from build123d import *

# Parameters (mm, degrees)
SKETCH1_W           = 47.117
SKETCH1_H           = 30.226
BOSS_EXTRUDE1_DEPTH = 23.8506
SKETCH4_W           = 44.069
SKETCH4_H           = 27.178
CUT_EXTRUDE1_DEPTH  = 61.847957117
SKETCH5_R           = 11.43
BOSS_EXTRUDE3_DEPTH = 44.069
SKETCH3_R           = 1.4986
CUT_EXTRUDE2_DEPTH  = 2.54
CUT_EXTRUDE3_START  = -2.54
SKETCH6_R           = 1.4986
CUT_EXTRUDE3_DEPTH  = 2.54
SKETCH2_R           = 1.4478
CUT_EXTRUDE4_DEPTH  = 61.847957117
SKETCH7_R           = 4.1783
CUT_EXTRUDE5_DEPTH  = 32.1564
CHAMFER1_SIZE       = 4.064
CHAMFER1_SIZE2      = 2.346351494


with BuildPart() as part:
    # Sketch1 → Boss-Extrude1 (new body)
    with BuildSketch(Plane.XY):
        with Locations((23.5585, 15.113)):
            Rectangle(SKETCH1_W, SKETCH1_H)
    extrude(amount=BOSS_EXTRUDE1_DEPTH)

    # Sketch4 → Cut-Extrude1 (cut, through all)
    with BuildSketch(Plane.XY.offset(23.8506)):
        with Locations((23.5585, 15.113)):
            Rectangle(SKETCH4_W, SKETCH4_H)
    extrude(amount=-CUT_EXTRUDE1_DEPTH, mode=Mode.SUBTRACT)

    # Sketch5 → Boss-Extrude3 (add)
    with BuildSketch(Plane(origin=(1.524, 0, 0), x_dir=(0, 0, -1), z_dir=(1, 0, 0))):
        with Locations(Location((-11.9253, 15.113, 0), (0, 0, 180))):
            Circle(SKETCH5_R)
    extrude(amount=BOSS_EXTRUDE3_DEPTH)

    # Sketch3 → Cut-Extrude2 (cut)
    with BuildSketch(Plane(origin=(0, 30.226, 0), x_dir=(1, 0, 0), z_dir=(0, 1, 0))):
        with Locations(Location((10.8585, -11.9253, 0), (0, 0, 270))):
            Circle(SKETCH3_R)
        with Locations(Location((36.2585, -11.9253, 0), (0, 0, 270))):
            Circle(SKETCH3_R)
    extrude(amount=-CUT_EXTRUDE2_DEPTH, mode=Mode.SUBTRACT)

    # Sketch6 → Cut-Extrude3 (cut)
    with BuildSketch(Plane.XZ.offset(CUT_EXTRUDE3_START)):
        with Locations(Location((15.9766, 19.812, 0), (0, 0, 270))):
            Circle(SKETCH6_R)
        with Locations(Location((10.8585, 11.9253, 0), (0, 0, 90))):
            Circle(SKETCH6_R)
        with Locations(Location((36.5506, 4.0386, 0), (0, 0, 270))):
            Circle(SKETCH6_R)
    extrude(amount=CUT_EXTRUDE3_DEPTH, mode=Mode.SUBTRACT)

    # Sketch2 → Cut-Extrude4 (cut, through all)
    with BuildSketch(Plane(origin=(47.117, 0, 0), x_dir=(0, 0, -1), z_dir=(1, 0, 0))):
        with Locations((-11.9253, 15.113)):
            Circle(SKETCH2_R)
    extrude(amount=-CUT_EXTRUDE4_DEPTH, mode=Mode.SUBTRACT)

    # Sketch7 → Cut-Extrude5 (cut)
    with BuildSketch(Plane.ZY):
        with Locations((11.9253, 15.113)):
            Circle(SKETCH7_R)
    extrude(amount=-CUT_EXTRUDE5_DEPTH, mode=Mode.SUBTRACT)

    # Chamfer1
    chamfer1_edges = [part.edges().sort_by_distance(p)[0] for p in [
        (32.1564, 15.113, 7.747),
    ]]
    chamfer1_side = [part.faces().sort_by_distance(p)[0] for p in [
        (16.0782, 15.113, 7.747),
    ]]
    chamfer(chamfer1_edges, length=CHAMFER1_SIZE, length2=CHAMFER1_SIZE2, reference=chamfer1_side[0])


solid = part.part
Part model, mm, in its own coordinate system. A direction names the side the tool comes from. Coordinates: 2 decimals unless noted, no trailing zeros. Order: outer loops, then holes, each group sorted by start corner. A loop starts at its lowest first (then second) coordinate and runs counter-clockwise, first axis right, second up. Notation, with made-up numbers: M 49.5,26.25 L 88.5,26.25 A20 cw 88.5,47.25 Z; hole C 62,-16.75 d2. An arc over 180 degrees is marked long. Use a Markdown table: item, result.
(1) Cut at D-D on z = 4.75. Write the cut outline in (x, y), then the cut area to 3 significant figures.
A:
| item | result |
|---|---|
| outline | M 0,0 L 35.23,0 L 35.23,1.52 L 1.52,1.52 L 1.52,6.22 L 45.59,6.22 L 45.59,1.52 L 37.87,1.52 L 37.87,0 L 47.12,0 L 47.12,30.23 L 0,30.23 Z; hole M 1.52,24.01 L 45.59,24.01 L 45.59,28.7 L 1.52,28.7 Z |
| area | 1,010 mm^2 |
(2) Pull direction Z, two halves, no side cores. Call faces 6 (the flat face through (23, 30.226, 12)), 7 (the flat face through (22, 1, 0)), 8 (the cylindrical face through (17.462, 0.773, 20.007)), 9 (the cylindrical face through (9.595, 0.773, 12.731)): released by +Z, released by -Z, zero draft, split by the parting line, or undercut.
A:
| item | result |
|---|---|
| face 6 | zero draft |
| face 7 | released by -Z |
| face 8 | undercut |
| face 9 | undercut |
(3) Cut at A-A on x = 33.5. Write the cut outline in (y, z).
A:
| item | result |
|---|---|
| outline | M 0,0 L 1.52,0 L 1.52,23.85 L 0,23.85 Z; C 15.11,11.93 d22.86; M 28.7,0 L 30.23,0 L 30.23,23.85 L 28.7,23.85 Z; hole C 15.11,11.93 d2.9 |
(4) Tool access for faces 1 (the cylindrical face through (10.285, 29.475, 13.31)), 2 (the cylindrical face through (23.25, 3.78, 10.44)), 3 (the cylindrical face through (35.088, 0.773, 4.363)), 4 (the flat face through (23, 28.702, 12)), 5 (the cylindrical face through (13.85, 17.94, 8.85)): list every direction of +Z, -Z, +X, -X, +Y, -Y with a clear straight run to the whole face (end or side of a thin tool).
A:
| item | result |
|---|---|
| face 1 | +Y |
| face 2 | none |
| face 3 | -Y |
| face 4 | +Z, -Z |
| face 5 | -X |
(5) Cut at C-C on z = 16.75. Write the cut outline in (x, y).
A:
| item | result |
|---|---|
| outline | M 0,0 L 47.12,0 L 47.12,30.23 L 0,30.23 Z; hole M 1.52,1.52 L 45.59,1.52 L 45.59,4.75 L 1.52,4.75 Z; hole M 1.52,25.47 L 45.59,25.47 L 45.59,28.7 L 1.52,28.7 Z |
(6) Flat gauge pins, fed straight in: pin 1 (2 mm diameter, centred on x = 42, y = 9, fed in from -Z); pin 2 (12 mm diameter, centred on x = 26.5, y = 14.5, fed in from +Z); pin 3 (10 mm diameter, centred on x = 36.5, y = 7.5, fed in from +Z). Where does each tip first touch, or does it go through?
A:
| item | result |
|---|---|
| pin 1 | stops at z = 1.7 |
| pin 2 | stops at z = 23.36 |
| pin 3 | stops at z = 23.05 |
(7) Cut at B-B on y = 27.5. Write the cut outline in (x, z).
A:
| item | result |
|---|---|
| outline | M 0,0 L 1.52,0 L 1.52,23.85 L 0,23.85 Z; M 45.59,0 L 47.12,0 L 47.12,23.85 L 45.59,23.85 Z |
(8) Probe L1, parallel to X at y = 5, z = 20.75; L2, parallel to Z at x = 35.5, y = 15; L3, parallel to Y at x = 34.5, z = 5.75. List the from-to ranges inside material, lowest first.
A:
| item | result |
|---|---|
| L1 | x = 0 to 1.52, 45.59 to 47.12 |
| L2 | z = 0.5 to 10.48, 13.37 to 23.35 |
| L3 | y = 0 to 1.52, 5.49 to 24.73, 28.7 to 30.23 |
